Here's how the part is built. I have some questions about the finished solid (model axes, mm). Give positions to 0.01 mm unless a question says otherwise; leave off trailing zeros. Loops run counter-clockwise (first coordinate to the right, second up) from the corner with the lowest first, then second, coordinate; pieces in that order, holes last.
Q1. I'm going to push a flat-ended pin straight in: P1, Ø8, axis at y = 149.5, z = 31, coming from the -X side. Where does the tip first touch, or does it pass through?
Q2. Thinking about a two-plate mould opening in Z: for faces 1 (the face through (-25, 321, -49.25)), 2 (the face through (-25, 321, 48.5)), 3 (the face through (-25, 321, 49.25)), 4 (the face through (0, 321, 1)), which applies, pulls with the +Z half, pulls with the -Z half, needs draft (parallel to the pull), parting line crosses it, or undercut?
Q3. Suppose I cut it at B-B (y = 458). List the corners of the cut face in (x, z) for me.
Q4. Suppose I cut it at C-C (z = -28). List the corners of the cut face in (x, y) for me.
Q5. I need wall thicknesses on probe 1 along Z at (x, y) = (-12, 512.5); probe 2 along X at (y, z) = (539.5, -40.5). Which ranges of each line are inside material? Lowest first, please.
Q6. Suppose I cut it at A-A (x = -7.5). List the corners of the cut face in (y, z) for me, and give its area (3 significant figures).
```python
from build123d import *

# Parameters (mm, degrees)
MOVE_BODY_2_DEPTH    = 3000
SKETCH_6_OUTSIDE_W   = 652.406
SKETCH_6_OUTSIDE_H   = 3602.406
SKETCH_6_OUTSIDE_W_2 = 50
SKETCH_6_OUTSIDE_H_2 = 650.75
CUT_EXTRUDE_1_DEPTH  = 3003.033019472


# Read off the part's stored shape, not the designer's step: Тело-Переместить/Копировать2
with BuildPart() as part:
    # Move Body 2 outline → Move Body 2 (new body)
    with BuildSketch(Plane(origin=(0, 0, 0), x_dir=(1, 0, 0), z_dir=(0, 1, 0))):
        with BuildLine():
            Line((-50, 47.75), (-50, 46.25))
            Line((-50, 46.25), (-49.25, 46.25))
            Line((-49.25, 46.25), (-49.25, 47.75))
            ThreePointArc((-49.25, 47.75), (-49.030330086, 48.280330086), (-48.5, 48.5))
            Line((-48.5, 48.5), (-1.5, 48.5))
            ThreePointArc((-1.5, 48.5), (-0.969669914, 48.280330086), (-0.75, 47.75))
            Line((-0.75, 47.75), (-0.75, -47.75))
            ThreePointArc((-0.75, -47.75), (-0.969669914, -48.280330086), (-1.5, -48.5))
            Line((-1.5, -48.5), (-48.5, -48.5))
            ThreePointArc((-48.5, -48.5), (-49.030330086, -48.280330086), (-49.25, -47.75))
            Line((-49.25, -47.75), (-49.25, -46.25))
            Line((-49.25, -46.25), (-50, -46.25))
            Line((-50, -46.25), (-50, -47.75))
            ThreePointArc((-50, -47.75), (-49.560660172, -48.810660172), (-48.5, -49.25))
            Line((-48.5, -49.25), (-1.5, -49.25))
            ThreePointArc((-1.5, -49.25), (-0.439339828, -48.810660172), (0, -47.75))
            Line((0, -47.75), (0, 47.75))
            ThreePointArc((0, 47.75), (-0.439339828, 48.810660172), (-1.5, 49.25))
            Line((-1.5, 49.25), (-48.5, 49.25))
            ThreePointArc((-48.5, 49.25), (-49.560660172, 48.810660172), (-50, 47.75))
        make_face()
    extrude(amount=MOVE_BODY_2_DEPTH)

    # Эскиз6 outside → Вырез-Вытянуть1 (cut, through all)
    with BuildSketch(Plane(origin=(0, 0, -49.25), x_dir=(-1, 0, 0), z_dir=(0, 0, -1))):
        with Locations((25, 1500)):
            Rectangle(SKETCH_6_OUTSIDE_W, SKETCH_6_OUTSIDE_H)
        with Locations((25, 325.375)):
            Rectangle(SKETCH_6_OUTSIDE_W_2, SKETCH_6_OUTSIDE_H_2, mode=Mode.SUBTRACT)
    extrude(amount=-CUT_EXTRUDE_1_DEPTH, mode=Mode.SUBTRACT)


solid = part.part
```
Solutions:
1. P1: stops at x = -0.75
2. face 1: pulls with the -Z half
2. face 2: undercut
2. face 3: pulls with the +Z half
2. face 4: needs draft
3. outline: (-50, -47.75) arc R1.5 ccw to (-48.5, -49.25) - (-1.5, -49.25) arc R1.5 ccw to (0, -47.75) - (0, 47.75) arc R1.5 ccw to (-1.5, 49.25) - (-48.5, 49.25) arc R1.5 ccw to (-50, 47.75) - (-50, 46.25) - (-49.25, 46.25) - (-49.25, 47.75) arc R0.75 cw to (-48.5, 48.5) - (-1.5, 48.5) arc R0.75 cw to (-0.75, 47.75) - (-0.75, -47.75) arc R0.75 cw to (-1.5, -48.5) - (-48.5, -48.5) arc R0.75 cw to (-49.25, -47.75) - (-49.25, -46.25) - (-50, -46.25) - close
4. outline: (-0.75, 0) - (0, 0) - (0, 650.75) - (-0.75, 650.75) - close
5. probe 1: z = -49.25 to -48.5, 48.5 to 49.25
5. probe 2: x = -0.75 to 0
6. outline: (0, -49.25) - (650.75, -49.25) - (650.75, -48.5) - (0, -48.5) - close; (0, 48.5) - (650.75, 48.5) - (650.75, 49.25) - (0, 49.25) - close
6. area: 976 mm2
